The model under review builds one solid part; all positions refer to its coordinate system, in mm. Face numbers are marked on the shaded views. Round coordinates to 2 decimals unless told otherwise and drop trailing zeros. Write each loop counter-clockwise with the first axis right and the second up, starting at its lowest first coordinate (ties: lowest second). Pieces come first, ordered by that corner, then holes.
Item 1: Add section D-D (x = -28.5). Give the boundary of the cut face in (y, z), plus the area to 3 significant figures.
Item 2: To check wall thickness, follow L1, parallel to Y at x = 0, z = -8.75; L2, parallel to Y at x = 0, z = 9.25; L3, parallel to X at y = -250, z = -8. State the ranges of each line that lie inside material, in increasing order.
Item 3: Draft analysis for pull direction Z (two halves, no side actions). For the marked faces 1, 2 and 3, state which applies: +Z half, -Z half, draft (parallel to the pull), parting line (faces both ways), or undercut.
Item 4: Clearance check with flat-ended pins moving along their axes: pin 1 Ø6 at (x, z) = (-14, 6) entering from +Y (3 decimals); pin 2 Ø8 at (x, z) = (7.5, -6) entering from -Y; pin 3 Ø3 at (x, z) = (-3, 0) entering from -Y; pin 4 Ø18 at (x, y) = (0, -250) entering from -Z. State where each tip first meets the part, or that it passes through.
Item 5: Add section B-B (x = 0). Give the boundary of the cut face in (y, z), plus the area to 3 significant figures.
Item 6: Add section A-A (z = 8.75). Give the boundary of the cut face in (x, y), plus the area to 3 significant figures.
Item 7: Add section C-C (y = -125). Give the boundary of the cut face in (x, z).
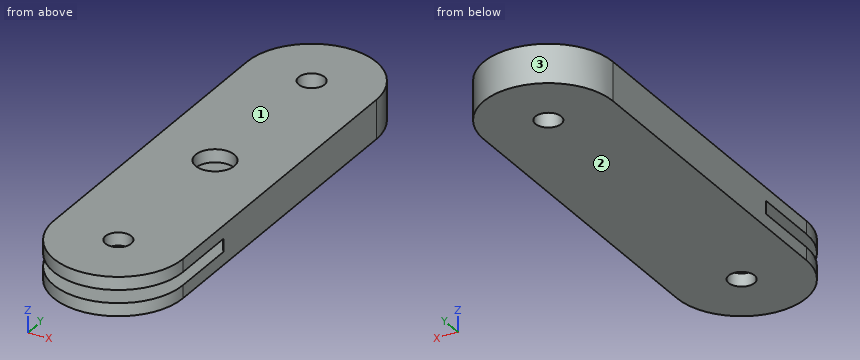
```python
from build123d import *

# Parameters (mm, degrees)
BOSS_EXTRU_2_DEPTH           = 15
ENL_V_MAT_EXTRU_1_DEPTH      = 5
ESQUISSE3_R                  = 10
ENL_V_MAT_EXTRU_2_DEPTH      = 306.614135799
ESQUISSE5_R                  = 15
ENL_V_MAT_EXTRU_3_DEPTH      = 15
ENL_V_MAT_EXTRU_4_DEPTH      = 210
ENL_V_MAT_EXTRU_4_DEPTH_BACK = 305.795013083
ESQUISSE4_R                  = 10


with BuildPart() as part:
    # Esquisse1 → Boss.-Extru.2 (new, symmetric)
    with BuildSketch(Plane.XY):
        with BuildLine():
            Line((50, 0), (50, -250))
            ThreePointArc((50, -250), (0, -300), (-50, -250))
            Line((-50, -250), (-50, 0))
            ThreePointArc((-50, 0), (0, 50), (50, 0))
        make_face()
    extrude(amount=BOSS_EXTRU_2_DEPTH, both=True)

    # Esquisse2 → Enlèv. mat.-Extru.1 (cut, symmetric)
    with BuildSketch(Plane.XY):
        with BuildLine():
            Line((44.95, -184.342455173), (44.95, -56.882832679))
            ThreePointArc((44.95, -56.882832679), (42.021067812, -49.811764867), (34.95, -46.882832679))
            Line((34.95, -46.882832679), (-34.95, -46.882832679))
            ThreePointArc((-34.95, -46.882832679), (-42.021067812, -49.811764867), (-44.95, -56.882832679))
            Line((-44.95, -56.882832679), (-44.95, -184.342455173))
            ThreePointArc((-44.95, -184.342455173), (-47.390043652, -193.91574787), (-54.114793306, -201.153115359))
            Line((-54.114793306, -201.153115359), (-50, -198.500950871))
            Line((-50, -198.500950871), (-50, -250))
            ThreePointArc((-50, -250), (0, -300), (50, -250))
            Line((50, -250), (50, -198.500950871))
            Line((50, -198.500950871), (54.114793306, -201.153115359))
            ThreePointArc((54.114793306, -201.153115359), (47.390043652, -193.91574787), (44.95, -184.342455173))
        make_face()
    extrude(amount=ENL_V_MAT_EXTRU_1_DEPTH, both=True, mode=Mode.SUBTRACT)

    # Esquisse3 → Enlèv. mat.-Extru.2 (cut, through all)
    with BuildSketch(Plane.XY.offset(15)):
        Circle(ESQUISSE3_R)
    extrude(amount=-ENL_V_MAT_EXTRU_2_DEPTH, mode=Mode.SUBTRACT)

    # Esquisse5 → Enlèv. mat.-Extru.3 (cut)
    with BuildSketch(Plane.XY.offset(15)):
        with Locations((0, -125)):
            Circle(ESQUISSE5_R)
    extrude(amount=-ENL_V_MAT_EXTRU_3_DEPTH, mode=Mode.SUBTRACT)

    # Esquisse4 → Enlèv. mat.-Extru.4 (cut, two sides: drawn at the far end of the back side and taken through both)
    with BuildSketch(Plane.XY.offset(-5).offset(-ENL_V_MAT_EXTRU_4_DEPTH_BACK)):
        with Locations((0, -250)):
            Circle(ESQUISSE4_R)
    extrude(amount=ENL_V_MAT_EXTRU_4_DEPTH + ENL_V_MAT_EXTRU_4_DEPTH_BACK, mode=Mode.SUBTRACT)


solid = part.part
```
Numbers:
1. outline: (-291.08, -15) - (41.08, -15) - (41.08, 15) - (-291.08, 15) - (-291.08, 5) - (-46.88, 5) - (-46.88, -5) - (-291.08, -5) - close
1. area: 7,520 mm2
2. L1: y = -300 to -260, -240 to -10, 10 to 50
2. L2: y = -300 to -260, -240 to -140, -110 to -10, 10 to 50
2. L3: x = -50 to -10, 10 to 50
3. face 1: +Z half
3. face 2: -Z half
3. face 3: draft
4. pin 1: stops at y = 48.775
4. pin 2: stops at y = -299.88
4. pin 3: stops at y = -46.88
4. pin 4: passes through
5. outline: (-300, -15) - (-260, -15) - (-260, -5) - (-300, -5) - close; (-300, 5) - (-260, 5) - (-260, 15) - (-300, 15) - close; (-240, -15) - (-10, -15) - (-10, 15) - (-110, 15) - (-110, 5) - (-46.88, 5) - (-46.88, -5) - (-240, -5) - close; (-240, 5) - (-140, 5) - (-140, 15) - (-240, 15) - close; (10, -15) - (50, -15) - (50, 15) - (10, 15) - close
5. area: 6,670 mm2
6. outline: (-50, -250) arc R50 ccw to (50, -250) - (50, 0) arc R50 ccw to (-50, 0) - close; hole circle Ø30 at (0, -125); hole circle Ø20 at (0, -250); hole circle Ø20 at (0, 0)
6. area: 31,500 mm2
7. outline: (-50, -15) - (50, -15) - (50, 15) - (15, 15) - (15, 5) - (44.95, 5) - (44.95, -5) - (-44.95, -5) - (-44.95, 5) - (-15, 5) - (-15, 15) - (-50, 15) - close
